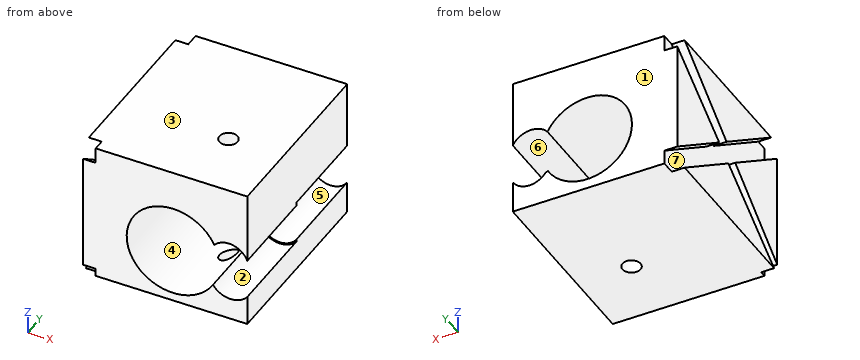
```python
from build123d import *

# Parameters (mm, degrees)
F0_W      = 54
F0_H      = 67
F0_R      = 3.2350840479
F1_DEPTH  = 50
F3_D      = 33
F3_DEPTH  = 33.0871826465
F4_D      = 32
F5_D      = 14
F5_DEPTH  = 33.0871827465
F6_D      = 14
F6_DEPTH  = 33.9148173535
F7_D      = 14
F7_DEPTH  = 33.0871827465
F8_D      = 15
F8_DEPTH  = 33.0871827465
F9_D      = 15
F10_D     = 15
F10_DEPTH = 33.9148173535
F12_DEPTH = 4.6


with BuildPart() as f1:
    # F0 (on Top) → F1 (new body)
    with BuildSketch(Plane.XY):
        with Locations((-9.3474117796, 0.4138173535)):
            Rectangle(F0_W, F0_H)
        with Locations((-1.7809633864, -9.1149061918)):
            Circle(F0_R, mode=Mode.SUBTRACT)
    extrude(amount=F1_DEPTH)

    # F3 (through all, one way)
    with BuildSketch(Plane(origin=(0, 0, 0), x_dir=(1, 0, 0), z_dir=(0, 1, 0))):
        with Locations((-8.8084321469, -19.4574296474)):
            Circle(F3_D / 2)
    extrude(amount=-F3_DEPTH, mode=Mode.SUBTRACT)

    # F4 (through all)
    with Locations(Plane.XZ):
        with Locations((-8.8084321469, 19.4574296474)):
            Hole(F4_D / 2)

    # F5 (through all, one way)
    with BuildSketch(Plane(origin=(0, 0, 0), x_dir=(1, 0, 0), z_dir=(0, 1, 0))):
        with Locations((11.1167700961, -22.2662836313)):
            Circle(F5_D / 2)
    extrude(amount=-F5_DEPTH, mode=Mode.SUBTRACT)

    # F6 (through all, one way)
    with BuildSketch(Plane.XZ):
        with Locations((11.7215663195, 15.209428966)):
            Circle(F6_D / 2)
    extrude(amount=-F6_DEPTH, mode=Mode.SUBTRACT)

    # F7 (through all, one way)
    with BuildSketch(Plane(origin=(0, 0, 0), x_dir=(1, 0, 0), z_dir=(0, 1, 0))):
        with Locations((7.8991507475, -18.4924459839)):
            Circle(F7_D / 2)
    extrude(amount=-F7_DEPTH, mode=Mode.SUBTRACT)

    # F8 (through all, one way)
    with BuildSketch(Plane(origin=(0, 0, 0), x_dir=(1, 0, 0), z_dir=(0, 1, 0))):
        with Locations((11.7215663195, -15.209428966)):
            Circle(F8_D / 2)
    extrude(amount=-F8_DEPTH, mode=Mode.SUBTRACT)

    # F9 (through all)
    with Locations(Plane.XZ):
        with Locations((7.8991507475, 18.4924459839)):
            Hole(F9_D / 2)

    # F10 (through all, one way)
    with BuildSketch(Plane.XZ):
        with Locations((11.1167700961, 22.2662836313)):
            Circle(F10_D / 2)
    extrude(amount=-F10_DEPTH, mode=Mode.SUBTRACT)

    # F11 (on face) → F12 (join)
    with BuildSketch(Plane(origin=(-36.3474117796, 0, 0), x_dir=(0, -1, 0), z_dir=(-1, 0, 0))):
        Polygon((-28.9854729855, 50), (-0.8816519102, 28.6277458975), (29.0403384715, 50), align=None)
        Polygon((-33.9138173535, 44.3356601551), (-33.9138173535, 5.0340001471), (-5.7946280701, 25.1185750987), align=None)
        Polygon((33.0861826465, 44.3356601551), (4.9187896518, 24.2166549416), (33.0861826465, 2.7960559819), align=None)
        Polygon((0.3256148099, 20.935907284), (-28.9854729855, 0), (30.959851897, 0), align=None)
    extrude(amount=F12_DEPTH)


solid = f1.part
```
Check sheet for the modelled part. Datum: model origin and axes. Units: mm. Face numbers are marked on the shaded views. A direction names the side the tool comes from. Coordinates: 2 decimals unless noted, no trailing zeros. Order: outer loops, then holes, each group sorted by start corner. A loop starts at its lowest first (then second) coordinate and runs counter-clockwise, first axis right, second up. Notation, with made-up numbers: (40.5, 52.5) -> (87.5, 52.5) arc R5 ccw to (87.5, 59.5) -> close; hole circle Ø8 at (22, -16.5). An arc over 180 degrees is marked (long way). Write item = value, one per line. Start each with the question number.
1) Access from +Z, -Z, +X, -X, +Y, -Y to the whole of each face (thin tool, end or side, straight path). Record for the marked faces 4, 5, 6 and 7.
2) Go/stop test with a flat-tipped pin: P1, Ø1.5, axis at y = 23.5, z = 9, coming from the -X side. Record where the tip stops, or that it passes through.
3) Material ranges on L1, parallel to Z at x = -38, y = 16.5; L2, parallel to Z at x = -37, y = -22; L3, parallel to X at y = -9, z = 10, recorded low to high.
4) Cross-section at A-A (x = 13). Enter the section's corners in (y, z).
5) Cross-section at D-D (x = -1). Enter the section's corners in (y, z).
6) Cross-section at C-C (z = 46.5). Enter the section's corners in (x, y).
7) Cross-section at B-B (y = -11.5). Enter the section's corners in (x, z), then the cut area to 3 significant figures.
8) Mould release check, pull along Z, two halves, no side actions. Record for the marked faces 1, 2 and 3: +Z half, -Z half, draft (parallel to the pull), parting line (faces both ways), or undercut.
Ans:
q1.face_4 = -Y
q1.face_5 = +Y, -Y
q1.face_6 = +Y
q1.face_7 = -X
q2.P1 = -36.35
q3.L1 = 0 to 8.92, 17.47 to 32.43, 40.51 to 50
q3.L2 = 0 to 6.12, 11.23 to 36.42, 44.97 to 50
q3.L3 = -40.95 to -22.33, 4.71 to 6.33, 17.12 to 17.65
q4.outline = (-33.09, 0) -> (33.91, 0) -> (33.91, 8.33) -> (0, 8.33) -> (0, 7.82) -> (-33.09, 7.82) -> close; (-33.09, 29.01) -> (0, 29.01) -> (0, 29.53) -> (33.91, 29.53) -> (33.91, 50) -> (-33.09, 50) -> close
q5.outline = (-33.09, 0) -> (-12.25, 0) -> (-12.25, 4.92) -> (-33.09, 4.92) -> close; (-33.09, 33.99) -> (-12.25, 33.99) -> (-12.25, 50) -> (-33.09, 50) -> close; (-5.98, 0) -> (33.91, 0) -> (33.91, 5.49) -> (0, 5.49) -> (0, 4.92) -> (-5.98, 4.92) -> close; (-5.98, 33.99) -> (0, 33.99) -> (0, 33.42) -> (33.91, 33.42) -> (33.91, 50) -> (-5.98, 50) -> close
q6.outline = (-40.95, -24.14) -> (-36.35, -24.14) -> (-36.35, -33.09) -> (17.65, -33.09) -> (17.65, 33.91) -> (-36.35, 33.91) -> (-36.35, 24.38) -> (-40.95, 24.38) -> close; hole circle Ø6.47 at (-1.78, -9.11)
q7.outline = (-40.95, 0) -> (-3.97, 0) -> (-3.97, 3.68) arc R16.5 cw (long way) to (-3.97, 35.23) -> (-3.97, 50) -> (-40.95, 50) -> (-40.95, 37.47) -> (-36.35, 37.47) -> (-36.35, 28.92) -> (-40.95, 28.92) -> (-40.95, 19.21) -> (-36.35, 19.21) -> (-36.35, 13.3) -> (-40.95, 13.3) -> close; (0.4, 0) -> (17.65, 0) -> (17.65, 10.62) arc R7.5 cw to (5.43, 11.12) arc R16.5 cw to (0.4, 5.77) -> close; (0.4, 33.15) arc R16.5 cw to (5.9, 26.93) arc R7 cw to (17.65, 24.77) -> (17.65, 50) -> (0.4, 50) -> close
q7.area = 1,710 mm²
q8.face_1 = draft
q8.face_2 = undercut
q8.face_3 = +Z half
